CAD build for the part. Positions are in the model's coordinates, mm. A direction names the side the tool comes from. Coordinates: 2 decimals unless noted, no trailing zeros. Order: outer loops, then holes, each group sorted by start corner. A loop starts at its lowest first (then second) coordinate and runs counter-clockwise, first axis right, second up. Notation, with made-up numbers: M 74,-10 L 117,-10 A20 cw 117,-1 Z; hole C 51.5,-30 d6. An arc over 180 degrees is marked long. One line per item, written item: value.
Autodesk Inventor part; units mm, degrees
ref_plane "YZ Plane" through (0, 0, 0) normal (1, 0, 0) x (0, 1, 0)
ref_plane "XZ Plane" through (0, 0, 0) normal (0, 1, 0) x (-1, 0, 0)
ref_plane "XY Plane" through (0, 0, 0) normal (0, 0, 1) x (1, 0, 0)
sketch "Sketch1" plane through (0, 0, 0) normal (0, 0, 1) x (1, 0, 0)
  line L0 (-101.6, -76.2) -> (101.6, -76.2)
  line L1 (101.6, -76.2) -> (101.6, 76.2)
  line L2 (101.6, 76.2) -> (-101.6, 76.2)
  line L3 (-101.6, 76.2) -> (-101.6, -76.2)
  line L4 (-101.6, -76.2) -> (101.6, 76.2) construction
  line L5 (101.6, -76.2) -> (-101.6, 76.2) construction
  point P0 (0, 0)
  dimension "d0" = 152.4
  dimension "d1" = 203.2
extrude "Extrusion1" add sketch "Sketch1" along normal blind 3.175
sketch "Sketch2" plane through (0, 0, 0) normal (0, 0, -1) x (-1, 0, 0)
  circle A0 centre (-37.1038, -82.4738) radius 101.092
  circle A1 centre (-37.1038, -82.4738) radius 107.442
  line L0 (-101.6, -76.2) -> (-101.6, 76.2)
  line L1 (-101.6, 3.4565) -> (-101.6, -76.2)
  line L2 (-101.6, -76.2) -> (70.1549, -76.2)
  line L3 (101.6, -76.2) -> (-101.6, -76.2)
  point P0 (0, 0)
  dimension "d4" = 214.884
extrude "Extrusion2" cut sketch "Sketch2" against normal blind 25.4 contours L2 L0 A0 | A0 L0 A1 L2 picked at (8.0579, -71.6086) picked at (67.4292, -71.4153)
fillet "Fillet1" radius 12.7 5 edges at (101.6, 76.2, 1.5875) (-101.6, 76.2, 1.5875) (-101.6, -76.2, 1.5875) (-70.1549, -76.2, 1.5875) (101.6, 3.4565, 1.5875)
sketch "Sketch3" plane through (0, 0, 0) normal (0, 0, -1) x (-1, 0, 0)
  line L0 (76.2027, 73.1012) -> (-660.4, 73.1012)
  line L1 (-660.4, 53.8988) -> (76.2027, 53.8988)
  circle A0 centre (-647.7, 63.5) radius 2.0701
  circle A1 centre (-622.3, 63.5) radius 2.0701
  circle A2 centre (-596.9, 63.5) radius 2.0701
  circle A3 centre (-571.5, 63.5) radius 2.0701
  circle A4 centre (-546.1, 63.5) radius 2.0701
  circle A5 centre (-520.7, 63.5) radius 2.0701
  circle A6 centre (-495.3, 63.5) radius 2.0701
  circle A7 centre (-469.9, 63.5) radius 2.0701
  circle A8 centre (-444.5, 63.5) radius 2.0701
  circle A9 centre (-419.1, 63.5) radius 2.0701
  circle A10 centre (-393.7, 63.5) radius 2.0701
  circle A11 centre (-368.3, 63.5) radius 2.0701
  circle A12 centre (-342.9, 63.5) radius 2.0701
  circle A13 centre (-317.5, 63.5) radius 2.0701
  circle A14 centre (-292.1, 63.5) radius 2.0701
  circle A15 centre (-266.7, 63.5) radius 2.0701
  circle A16 centre (-241.3, 63.5) radius 2.0701
  circle A17 centre (-215.9, 63.5) radius 2.0701
  circle A18 centre (-190.5, 63.5) radius 2.0701
  circle A19 centre (-165.1, 63.5) radius 2.0701
  circle A20 centre (-139.7, 63.5) radius 2.0701
  circle A21 centre (-114.3, 63.5) radius 2.0701
  circle A22 centre (-88.9, 63.5) radius 2.0701
  circle A23 centre (-63.5, 63.5) radius 2.0701
  circle A24 centre (-38.1, 63.5) radius 2.0701
  circle A25 centre (-12.7, 63.5) radius 2.0701
  circle A26 centre (12.7, 63.5) radius 2.0701
  circle A27 centre (38.1, 63.5) radius 2.0701
  circle A28 centre (63.5, 63.5) radius 2.0701
  line L2 (97.2058, -44.2468) -> (78.359, -44.2468)
  line L3 (78.359, -44.2468) -> (76.2, -42.0878)
  line L4 (76.2, 16.8402) -> (76.2, -42.0878)
  line L5 (76.2, 16.8402) -> (78.359, 18.9992)
  line L6 (97.2058, 18.9992) -> (78.359, 18.9992)
  line L7 (97.2058, -44.2468) -> (97.2058, 18.9992)
  circle A29 centre (88.9, 12.7762) radius 2.0701
  circle A30 centre (88.9, 0.0762) radius 2.0701
  circle A31 centre (88.9, -12.6238) radius 2.0701
  circle A32 centre (88.9, -25.3238) radius 2.0701
  circle A33 centre (88.9, -38.0238) radius 2.0701
  line L8 (76.2027, 73.1012) -> (76.2027, 53.8988)
  line L9 (-660.4, 53.8988) -> (-660.4, 73.1012)
  point P0 (0, 0)
  point P1 (88.9, 25.4762)
  point P2 (88.9, 38.1762)
  dimension "d17" = 12.7
hole "Hole1" at (88.9, 63.5, 0) at (63.5, 63.5, 0) at (38.1, 63.5, 0) at (12.7, 63.5, 0) at (-12.7, 63.5, 0) at (-38.1, 63.5, 0) at (-63.5, 63.5, 0) at (-88.9, 12.7762, 0) at (-88.9, 0.0762, 0) at (-88.9, -12.6238, 0) at (-88.9, -25.3238, 0) at (-88.9, -38.0238, 0) at (-88.9, 25.4762, 0) at (-88.9, 38.1762, 0) direction (0, 0, 1) diameter 4.1402 end through all
sketch "Sketch4" plane through (0, 0, 0) normal (0, 0, -1) x (-1, 0, 0)
  line L0 (-88.9, 76.2) -> (88.9, 76.2)
  line L1 (-25.4, 76.2) -> (25.4, 76.2)
  line L2 (25.4, 76.2) -> (25.4, 44.45)
  line L3 (25.4, 44.45) -> (-25.4, 44.45)
  line L4 (-25.4, 44.45) -> (-25.4, 76.2)
  line L5 (-101.6, 25.9294) -> (-101.6, 63.5)
  point P0 (0, 0)
  dimension "d23" = 31.75
  dimension "d24" = 50.8
  dimension "d25" = 76.2
extrude "Extrusion3" cut sketch "Sketch4" against normal through all
fillet "Fillet2" radius 12.7 4 edges at (25.4, 76.2, 1.5875) (25.4, 44.45, 1.5875) (-25.4, 44.45, 1.5875) (-25.4, 76.2, 1.5875)
properties part number "C13_TK_UpperFrameSupportWheel" material "Polycarbonate, Clear"
Q1. Slice it at B-B (z = 1.45). Give the number of separate pieces and of enclosed holes in the cut face, plus the area to 3 significant figures.
Recorded:
separate pieces: 1
enclosed holes: 12
area: 14,500 mm^2
Q2. Drill centre lines: line 1 along X through (y, z) = (60, 2.45); line 2 along X through (y, z) = (-14, 1.8); line 3 along Y through (x, z) = (-14, 1.85). Where is each one in solid material? Low to high.
Recorded:
line 1: x = -101.6 to -25.4, 25.4 to 101.6
line 2: x = -101.6 to -90.45, -87.35 to -45.69
line 3: y = 12.04 to 44.52
Q3. Which spindle directions (+Z, -Z, +X, -X, +Y, -Y) get a long thin tool onto all of the face, cutting with end or side? Do faces 1 (the face through (37.478, 65.475, 1.61)), 2 (the face through (-29.02, 72.38, 1.61)). Say none if no direction does.
Recorded:
face 1: +Z, -Z
face 2: +Z, -Z, +Y
Q4. Pin check, flat tips, straight feed: pin 1 Ø1 at (x, z) = (3, 2) entering from +Y; pin 2 Ø1.5 at (y, z) = (-44, 0.5) entering from +X. Stop position of each tip, or through.
Recorded:
pin 1: stops at y = 44.45
pin 2: stops at x = -62.92
Q5. Slice it at C-C (y = 54). List the corners of the cut face in (x, z) (3 decimals).
Recorded:
outline: M -101.6,0 L -25.003,0 L -25.003,3.175 L -101.6,3.175 Z; M 25.003,0 L 101.6,0 L 101.6,3.175 L 25.003,3.175 Z
Q6. Slice it at A-A (x = 63.5). List the corners of the cut face in (y, z) (3 decimals).
Recorded:
outline: M 21.675,0 L 61.43,0 L 61.43,3.175 L 21.675,3.175 Z; M 65.57,0 L 76.2,0 L 76.2,3.175 L 65.57,3.175 Z
Q7. Mould opens along Y. For faces 3 (the face through (-97.98, -72.38, 1.61)), 4 (the face through (21.58, 48.07, 1.61)), 5 (the face through (-64.122, 65.475, 1.61)), 6 (the face through (-24, 18, 3.175)) say: released by +Y, released by -Y, zero draft, split by the parting line, or undercut.
Recorded:
face 3: released by -Y
face 4: released by +Y
face 5: undercut
face 6: zero draft
